Autodesk Inventor part; units mm, degrees
ref_plane "作業平面1" through (0, 0, 0) normal (0, 1, 0) x (-1, 0, 0)
ref_plane "YZ Plane" through (0, 0, 0) normal (1, 0, 0) x (0, 1, 0)
ref_plane "XY Plane" through (0, 0, 0) normal (0, 0, 1) x (1, 0, 0)
sketch "スケッチ1" plane through (0, 0, 0) normal (0, 0, 1) x (1, 0, 0)
  circle A0 centre (0, 0) radius 13.6
  dimension "d0" = 27.2
extrude "押し出し1" add sketch "スケッチ1" against normal blind 450
sketch "スケッチ3" plane through (0, 0, 0) normal (0, 0, 1) x (1, 0, 0)
  circle A0 centre (0, 0) radius 13.6
hole "穴1" at (0, 0, 0) direction (0, 0, -1) diameter 22.6 end through all
ref_plane "作業平面1" through (0, 0, 0) normal (0, 1, 0) x (-1, 0, 0)
sketch "スケッチ4" plane through (0, 0, 0) normal (0, 1, 0) x (-1, 0, 0)
  line L0 (-13.6, 0) -> (13.6, 0)
  arc A0 (-13.6, 0) -> (13.6, 0) centre (0, 0) ccw
  line L1 (13.6, 0) -> (-13.6, 0)
extrude "押し出し3" cut sketch "スケッチ4" along normal mid plane 27.2
sketch "スケッチ5" plane through (0, 0, 0) normal (0, 1, 0) x (-1, 0, 0)
  line L0 (-13.6, -450) -> (13.6, -450)
  arc A0 (13.6, -450) -> (-13.6, -450) centre (0, -450) ccw
  line L1 (-13.6, -450) -> (13.6, -450)
  point P0 (0, 0)
extrude "押し出し4" cut sketch "スケッチ5" along normal mid plane 27.2
properties part number "縦のパイプ"
Design review of the part built by this model. Coordinates are the model's own, in mm. Round coordinates to 2 decimals unless told otherwise and drop trailing zeros. Write each loop counter-clockwise with the first axis right and the second up, starting at its lowest first coordinate (ties: lowest second). Pieces come first, ordered by that corner, then holes. Notation, with made-up numbers: M 57,70.5 L 65,70.5 A19 cw 65,87.5 Z; hole C -9.5,4.25 d6. An arc over 180 degrees is marked long. One line per item, written item: value. Start each with the question number.
1. Take a section at C-C on z = -230. State the section outline as (x, y) points, then the cut area to 3 significant figures.
2. To check wall thickness, follow probe 1 along X at (y, z) = (0, -281); probe 2 along X at (y, z) = (-1.25, -355). State the ranges of each line that lie inside material, in increasing order. Write a range as from..to.
3. Draft analysis for pull direction X (two halves, no side actions). For faces 1 (the face through (-2.948, -13.277, -221.85)), 2 (the face through (-3.39, -10.78, -228.04)), state which applies: pulls with the +X half, pulls with the -X half, needs draft (parallel to the pull), parting line crosses it, or undercut.
4. Clearance check with flat-ended pins moving along their axes: P1, Ø8, axis at y = 9.5, z = -74, coming from the -X side; P2, Ø5, axis at y = 3.5, z = -235, coming from the +X side; P3, Ø6, axis at x = -5, z = -237.5, coming from the +Y side. State where each tip first meets the part, or that it passes through.
5. Take a section at A-A on x = 0. State the section outline as (y, z) points.
6. Take a section at B-B on y = 0. State the section outline as (x, z) points.
Computed:
1. outline: C 0,0 d27.2; hole C 0,0 d22.6
1. area: 180 mm²
2. probe 1: x = -13.6..-11.3, 11.3..13.6
2. probe 2: x = -13.54..-11.23, 11.23..13.54
3. face 1: parting line crosses it
3. face 2: undercut
4. P1: stops at x = -12.44
4. P2: stops at x = 13.56
4. P3: stops at y = 13.45
5. outline: M -13.6,-436.4 L -11.3,-436.4 L -11.3,-13.6 L -13.6,-13.6 Z; M 11.3,-436.4 L 13.6,-436.4 L 13.6,-13.6 L 11.3,-13.6 Z
6. outline: M -13.6,-450 A13.6 cw -11.3,-442.43 L -11.3,-7.57 A13.6 cw -13.6,0 Z; M 11.3,-442.43 A13.6 cw 13.6,-450 L 13.6,0 A13.6 cw 11.3,-7.57 Z
